Drawing for the job (mm, zero at the part's lowest x, y, z). A direction names the side the tool comes from. Give positions to 0.01 mm unless a question says otherwise; leave off trailing zeros. Order: outer loops, then holes, each group sorted by start corner. A loop starts at its lowest first (then second) coordinate and runs counter-clockwise, first axis right, second up. Notation, with made-up numbers: (22, -1.75) - (67, -1.75) arc R24 cw to (67, 15.25) - close; hole circle Ø1 at (12, -36.5). An arc over 180 degrees is marked (long way). Use a Markdown table: item, result.
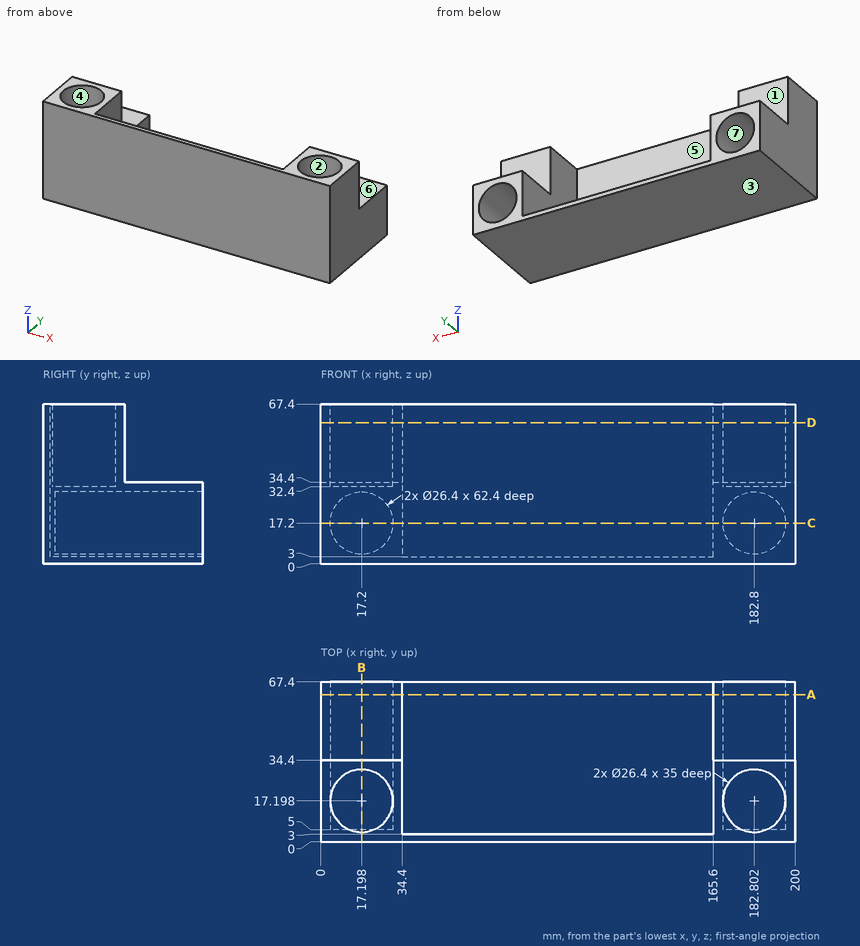
1) Tool access for the marked faces 5, 6 and 7: list every direction of +Z, -Z, +X, -X, +Y, -Y with a clear straight run to the whole face (end or side of a thin tool).
Computed:
| item | result |
|---|---|
| face 5 | +Z, +Y |
| face 6 | +Z, +X, -X, +Y |
| face 7 | +Y |
2) Pin check, flat tips, straight feed: P1, Ø12, axis at x = 67.5, y = 32.5, coming from the +Z side; P2, Ø13, axis at x = 188, y = 13.5, coming from the +Z side; P3, Ø13, axis at x = 177, z = 17.5, coming from the +Y side. Stop position of each tip, or through.
Computed:
| item | result |
|---|---|
| P1 | stops at z = 3 |
| P2 | stops at z = 32.4 |
| P3 | stops at y = 5 |
3) Slice it at C-C (z = 17.2). Write the cut outline in (x, y).
Computed:
| item | result |
|---|---|
| outline | (0, 0) - (200, 0) - (200, 67.4) - (196, 67.4) - (196, 5) - (169.6, 5) - (169.6, 67.4) - (165.6, 67.4) - (165.6, 3) - (34.4, 3) - (34.4, 67.4) - (30.4, 67.4) - (30.4, 5) - (4, 5) - (4, 67.4) - (0, 67.4) - close |
4) Two-plate mould, pull along Y, no slides. Class the marked faces 1, 2, 3 and 4: +Y half, -Y half, draft (parallel to the pull), parting line (faces both ways), or undercut.
Computed:
| item | result |
|---|---|
| face 1 | +Y half |
| face 2 | undercut |
| face 3 | draft |
| face 4 | undercut |
5) Wall check: line 1 (X direction, y = 46, z = 17); line 2 (X direction, y = 15, z = 60) (1 decimal); line 3 (X direction, y = 33.5, z = 64). Give the ranges that are in metal, low to high. Write a range as from..to.
Computed:
| item | result |
|---|---|
| line 1 | x = 0..4, 30.4..34.4, 165.6..169.6, 196..200 |
| line 2 | x = 0..4.2, 30.2..34.4, 165.6..169.8, 195.8..200 |
| line 3 | x = 0..34.4, 165.6..200 |
6) Slice it at B-B (x = 17.2). Write the cut outline in (y, z).
Computed:
| item | result |
|---|---|
| outline | (0, 0) - (67.4, 0) - (67.4, 4) - (5, 4) - (5, 30.4) - (67.4, 30.4) - (67.4, 34.4) - (34.4, 34.4) - (34.4, 67.4) - (30.4, 67.4) - (30.4, 32.4) - (4, 32.4) - (4, 67.4) - (0, 67.4) - close |
7) Slice it at A-A (y = 62). Write the cut outline in (x, z).
Computed:
| item | result |
|---|---|
| outline | (0, 0) - (200, 0) - (200, 34.4) - (165.6, 34.4) - (165.6, 3) - (34.4, 3) - (34.4, 34.4) - (0, 34.4) - close; hole circle Ø26.4 at (17.2, 17.2); hole circle Ø26.4 at (182.8, 17.2) |
